For this review, use the dimensioned drawing (mm, ordinates from the lowest corner) and the shaded views. Coordinates: 2 decimals unless noted, no trailing zeros. Write each loop counter-clockwise with the first axis right and the second up, starting at its lowest first coordinate (ties: lowest second). Pieces come first, ordered by that corner, then holes. Notation, with made-up numbers: M 60,70.25 L 86,70.25 A21 cw 86,75.25 Z; hole C 47,-5.5 d6. An arc over 180 degrees is marked long. One line per question, with ' | ' between items.
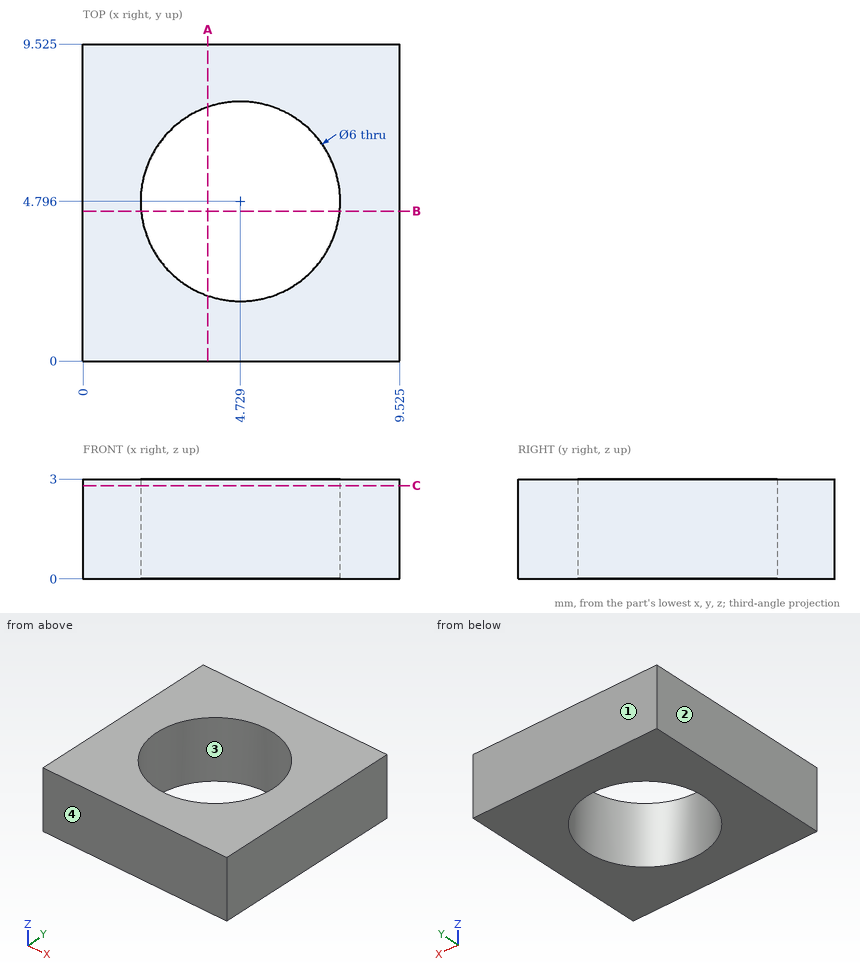
1. Take a section at A-A (x = 3.75). Write out the cut boundary in (y, z) (1 decimal).
Answer sheet:
outline: M 0,0 L 2,0 L 2,3 L 0,3 Z; M 7.6,0 L 9.5,0 L 9.5,3 L 7.6,3 Z
2. Take a section at B-B (y = 4.5). Write out the cut boundary in (x, z) (1 decimal).
Answer sheet:
outline: M 0,0 L 1.7,0 L 1.7,3 L 0,3 Z; M 7.7,0 L 9.5,0 L 9.5,3 L 7.7,3 Z
3. Take a section at C-C (z = 2.8). Write out the cut boundary in (x, y) (1 decimal).
Answer sheet:
outline: M 0,0 L 9.5,0 L 9.5,9.5 L 0,9.5 Z; hole C 4.7,4.8 d6
4. To check wall thickness, follow line 1 along Y through (x, z) = (4.75, 1.6) (1 decimal); line 2 along Y through (x, z) = (6, 1.85) (1 decimal); line 3 along X through (y, z) = (7.5, 1.3) (1 decimal). State the ranges of each line that lie inside material, in increasing order. Write a range as [from, to].
Answer sheet:
line 1: [0, 1.8], [7.8, 9.5] | line 2: [0, 2.1], [7.5, 9.5] | line 3: [0, 3.4], [6, 9.5]
5. Draft analysis for pull direction Y (two halves, no side actions). For the marked faces 1, 2, 3 and 4, state which applies: pulls with the +Y half, pulls with the -Y half, needs draft (parallel to the pull), parting line crosses it, or undercut.
Answer sheet:
face 1: pulls with the +Y half | face 2: needs draft | face 3: undercut | face 4: pulls with the -Y half
